from build123d import *

# Parameters (mm, degrees)
EXTRUDE_1_DEPTH     = 50
CUT_EXTRUDE_1_DEPTH = 13
CUT_EXTRUDE_2_DEPTH = 27
CUT_EXTRUDE_3_DEPTH = 50


with BuildPart() as part:
    # Sketch 1 → Extrude 1 (new body)
    with BuildSketch(Plane(origin=(0, 0, 0), x_dir=(1, 0, 0), z_dir=(0, 1, 0))):
        Polygon((0, 0), (654, 0), (654.0000000000001, -960), (1.1757e-13, -960), align=None)
    extrude(amount=-EXTRUDE_1_DEPTH)

    # Sketch 1_4 → Cut-Extrude 1 (cut)
    with BuildSketch(Plane(origin=(0, 0, 0), x_dir=(1, 0, 0), z_dir=(0, 1, 0))):
        with BuildLine():
            Line((5.0000000000000355, -275), (5.0000000000000355, -244.9999999999999))
            ThreePointArc((5.0000000000000355, -244.9999999999999), (10.857864376269086, -230.85786437626894), (25.000000000000036, -224.99999999999986))
            Line((25.000000000000036, -224.99999999999986), (574.9999999999997, -224.99999999999986))
            ThreePointArc((574.9999999999997, -224.99999999999986), (599.748737341529, -235.2512626584707), (609.9999999999999, -260.0000000000001))
            Line((609.9999999999999, -260.0000000000001), (609.9999999999999, -369.9999999999998))
            ThreePointArc((609.9999999999999, -369.9999999999998), (599.748737341529, -394.7487373415292), (574.9999999999997, -405))
            Line((574.9999999999997, -405), (110.0000000000001, -405.00000000000006))
            Line((110.0000000000001, -405.00000000000006), (110.00000000000007, -444.9999999999999))
            Line((110.00000000000007, -444.9999999999999), (574.9999999999998, -444.99999999999966))
            ThreePointArc((574.9999999999998, -444.99999999999966), (599.7487373415292, -455.2512626584705), (610, -479.99999999999994))
            Line((610, -479.99999999999994), (610, -589.9999999999995))
            ThreePointArc((610, -589.9999999999995), (599.7487373415291, -614.7487373415289), (574.9999999999998, -624.9999999999998))
            Line((574.9999999999998, -624.9999999999998), (110.0000000000001, -625))
            Line((110.0000000000001, -625), (110.00000000000011, -665.0000000000001))
            Line((110.00000000000011, -665.0000000000001), (625.0000000000001, -665.0000000000002))
            ThreePointArc((625.0000000000001, -665.0000000000002), (639.142135623731, -670.8578643762693), (645.0000000000001, -685.0000000000001))
            Line((645.0000000000001, -685.0000000000001), (645.0000000000001, -714.9999999999998))
            ThreePointArc((645.0000000000001, -714.9999999999998), (639.1421356237311, -729.1421356237307), (625.0000000000001, -734.9999999999997))
            Line((625.0000000000001, -734.9999999999997), (75.0000000000004, -734.9999999999999))
            ThreePointArc((75.0000000000004, -734.9999999999999), (50.25126265847098, -724.748737341529), (40.000000000000135, -699.9999999999997))
            Line((40.000000000000135, -699.9999999999997), (40.0000000000001, -590.0000000000001))
            ThreePointArc((40.0000000000001, -590.0000000000001), (50.25126265847094, -565.2512626584708), (75.00000000000034, -554.9999999999998))
            Line((75.00000000000034, -554.9999999999998), (539.9999999999999, -554.9999999999998))
            Line((539.9999999999999, -554.9999999999998), (539.9999999999999, -514.9999999999997))
            Line((539.9999999999999, -514.9999999999997), (75.00000000000036, -515))
            ThreePointArc((75.00000000000036, -515), (50.251262658470964, -504.7487373415292), (40.000000000000085, -479.9999999999998))
            Line((40.000000000000085, -479.9999999999998), (40.00000000000005, -370.0000000000004))
            ThreePointArc((40.00000000000005, -370.0000000000004), (50.25126265847087, -345.251262658471), (75.00000000000028, -335.0000000000001))
            Line((75.00000000000028, -335.0000000000001), (540, -335))
            Line((540, -335), (540, -295.00000000000006))
            Line((540, -295.00000000000006), (25.000000000000036, -295.00000000000006))
            ThreePointArc((25.000000000000036, -295.00000000000006), (10.857864376269081, -289.14213562373095), (5.0000000000000355, -275))
        make_face()
    extrude(amount=-CUT_EXTRUDE_1_DEPTH, mode=Mode.SUBTRACT)

    # Sketch 1_5 → Cut-Extrude 2 (cut)
    with BuildSketch(Plane(origin=(0, 0, 0), x_dir=(1, 0, 0), z_dir=(0, 1, 0))):
        with BuildLine():
            Line((25.00000000000002, -229.99999999999986), (574.9999999999999, -229.99999999999983))
            ThreePointArc((574.9999999999999, -229.99999999999983), (596.2132034355964, -238.78679656440343), (604.9999999999999, -259.9999999999999))
            Line((604.9999999999999, -259.9999999999999), (604.9999999999999, -370))
            ThreePointArc((604.9999999999999, -370), (596.2132034355964, -391.2132034355964), (574.9999999999999, -400))
            Line((574.9999999999999, -400), (105.00000000000007, -400.00000000000006))
            Line((105.00000000000007, -400.00000000000006), (105.00000000000007, -449.9999999999999))
            Line((105.00000000000007, -449.9999999999999), (575, -449.99999999999966))
            ThreePointArc((575, -449.99999999999966), (596.2132034355964, -458.78679656440323), (605, -479.99999999999966))
            Line((605, -479.99999999999966), (605, -589.9999999999998))
            ThreePointArc((605, -589.9999999999998), (596.2132034355964, -611.2132034355961), (575, -619.9999999999998))
            Line((575, -619.9999999999998), (105.00000000000011, -620))
            Line((105.00000000000011, -620), (105.00000000000011, -670.0000000000001))
            Line((105.00000000000011, -670.0000000000001), (625, -670.0000000000001))
            ThreePointArc((625, -670.0000000000001), (635.6066017177983, -674.3933982822019), (640.0000000000001, -685.0000000000002))
            Line((640.0000000000001, -685.0000000000002), (640.0000000000001, -714.9999999999997))
            ThreePointArc((640.0000000000001, -714.9999999999997), (635.6066017177983, -725.606601717798), (625, -729.9999999999998))
            Line((625, -729.9999999999998), (75.00000000000007, -730))
            ThreePointArc((75.00000000000007, -730), (53.786796564403645, -721.2132034355964), (45.00000000000012, -700))
            Line((45.00000000000012, -700), (45.00000000000009, -589.9999999999999))
            ThreePointArc((45.00000000000009, -589.9999999999999), (53.78679656440367, -568.7867965644034), (75.00000000000009, -559.9999999999999))
            Line((75.00000000000009, -559.9999999999999), (544.9999999999999, -559.9999999999998))
            Line((544.9999999999999, -559.9999999999998), (544.9999999999999, -509.99999999999966))
            Line((544.9999999999999, -509.99999999999966), (75.00000000000009, -510))
            ThreePointArc((75.00000000000009, -510), (53.786796564403616, -501.2132034355964), (45.00000000000007, -479.99999999999994))
            Line((45.00000000000007, -479.99999999999994), (45.00000000000004, -370.0000000000001))
            ThreePointArc((45.00000000000004, -370.0000000000001), (53.786796564403616, -348.7867965644037), (75.00000000000003, -340.00000000000006))
            Line((75.00000000000003, -340.00000000000006), (545, -340))
            Line((545, -340), (545, -290.00000000000006))
            Line((545, -290.00000000000006), (25.00000000000002, -290.00000000000006))
            ThreePointArc((25.00000000000002, -290.00000000000006), (14.393398282201769, -285.60660171779824), (10.000000000000036, -275))
            Line((10.000000000000036, -275), (10.000000000000036, -244.9999999999999))
            ThreePointArc((10.000000000000036, -244.9999999999999), (14.393398282201789, -234.39339828220164), (25.00000000000002, -229.99999999999986))
        make_face()
    extrude(amount=-CUT_EXTRUDE_2_DEPTH, mode=Mode.SUBTRACT)

    # Sketch 1_6 → Cut-Extrude 3 (cut)
    with BuildSketch(Plane(origin=(0, 0, 0), x_dir=(1, 0, 0), z_dir=(0, 1, 0))):
        with BuildLine():
            ThreePointArc((10.000000000000018, -275), (10.052542158175607, -276.2543939041952), (10.20980054225095, -277.4999999999999))
            Line((10.20980054225095, -277.49999999999994), (35.00000000000021, -277.49999999999994))
            ThreePointArc((35.00000000000021, -277.49999999999994), (38.53553390593298, -276.03553390593265), (40.000000000000256, -272.4999999999999))
            Line((40.00000000000024, -272.4999999999999), (40.00000000000024, -247.5))
            ThreePointArc((40.00000000000024, -247.5), (38.53553390593298, -243.96446609406723), (35.00000000000021, -242.49999999999997))
            Line((35.00000000000021, -242.49999999999997), (10.209800542250957, -242.49999999999997))
            ThreePointArc((10.209800542250964, -242.5), (10.052542158175624, -243.7456060958047), (10.000000000000037, -244.9999999999999))
            Line((10.000000000000036, -244.9999999999999), (10.000000000000036, -275))
        make_face()
        with BuildLine():
            Line((610.0000000000002, -712.5), (610.0000000000002, -687.5))
            ThreePointArc((610.0000000000002, -687.5), (611.4644660940675, -683.9644660940672), (615.0000000000002, -682.5))
            Line((615.0000000000002, -682.5), (640.0000000000002, -682.5))
            ThreePointArc((640.0000000000002, -682.5), (643.535533905933, -683.9644660940672), (645.0000000000002, -687.5))
            Line((645.0000000000002, -687.5), (645.0000000000002, -712.5))
            ThreePointArc((645.0000000000002, -712.5), (643.535533905933, -716.0355339059328), (640.0000000000002, -717.5))
            Line((640.0000000000002, -717.5), (615.0000000000002, -717.5))
            ThreePointArc((615.0000000000002, -717.5), (611.4644660940675, -716.0355339059328), (610.0000000000002, -712.5))
        make_face()
    extrude(amount=-CUT_EXTRUDE_3_DEPTH, mode=Mode.SUBTRACT)


solid = part.part
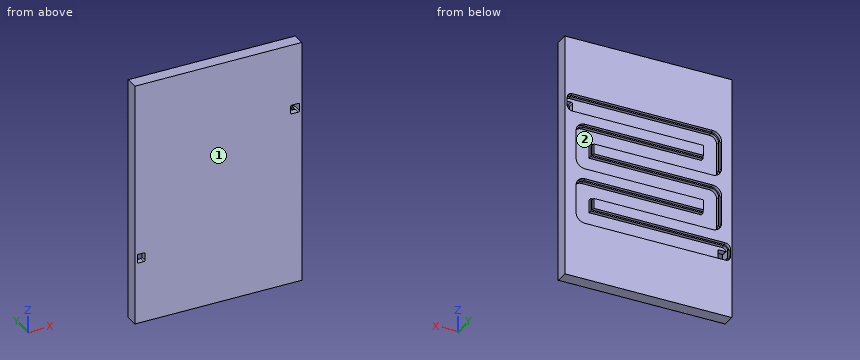
Can you work these out from the model? Positions are in its coordinate system, mm. Face numbers are marked on the shaded views. Coordinates: 2 decimals unless noted, no trailing zeros. Write each loop counter-clockwise with the first axis right and the second up, starting at its lowest first coordinate (ties: lowest second). Pieces come first, ordered by that corner, then holes. Notation, with made-up numbers: (88.5, -32) - (94.5, -32) arc R34 ccw to (94.5, -1) - close; hole circle Ø3 at (41.5, 46.25). An arc over 180 degrees is marked (long way). Return JSON: item names as keys, results as strings. Group by question number.
Item 1: Please list where these lines run through material, in increasing order: probe 1 along Z at (x, y) = (85, -4.5); probe 2 along Z at (x, y) = (562, -23); probe 3 along Z at (x, y) = (404.5, -4.5).
Item 2: If we section it at A-A (z = 639): Write out the boundary of the cut face in (x, y), then the cut area to 4 significant figures.
Item 3: We'd pull the mould along X, two halves only. Please class the marked faces 1 and 2: pulls with the +X half, pulls with the -X half, needs draft (parallel to the pull), parting line crosses it, or undercut.
Item 4: If we section it at C-C (z = 467.5): Write out the boundary of the cut face in (x, y).
Item 5: If we section it at B-B (x = 65): Write out the boundary of the cut face in (y, z).
Return value:
{
 "1": {"probe 1": "z = 0 to 225, 295 to 335, 515 to 555, 735 to 960", "probe 2": "z = 0 to 230, 400 to 450, 620 to 670, 730 to 960", "probe 3": "z = 0 to 225, 295 to 335, 405 to 445, 515 to 555, 625 to 665, 735 to 960"},
 "2": {"outline": "(0, -50) - (654, -50) - (654, 0) - (110, 0) - (110, -13) - (105, -13) - (105, -27) - (45, -27) - (45, -13) - (40, -13) - (40, 0) - (0, 0) - close", "area": "30,950 mm^2"},
 "3": {"face 1": "needs draft", "face 2": "undercut"},
 "4": {"outline": "(0, -50) - (654, -50) - (654, 0) - (607.69, 0) - (607.69, -13) - (602.27, -13) - (602.27, -27) - (45, -27) - (45, -13) - (40, -13) - (40, 0) - (0, 0) - close"},
 "5": {"outline": "(-50, 0) - (0, 0) - (0, 225) - (-13, 225) - (-13, 230) - (-27, 230) - (-27, 290) - (-13, 290) - (-13, 295) - (0, 295) - (0, 336.46) - (-13, 336.46) - (-13, 341.72) - (-27, 341.72) - (-27, 508.28) - (-13, 508.28) - (-13, 513.54) - (0, 513.54) - (0, 556.46) - (-13, 556.46) - (-13, 561.72) - (-27, 561.72) - (-27, 728.28) - (-13, 728.28) - (-13, 733.54) - (0, 733.54) - (0, 960) - (-50, 960) - close"}
}
